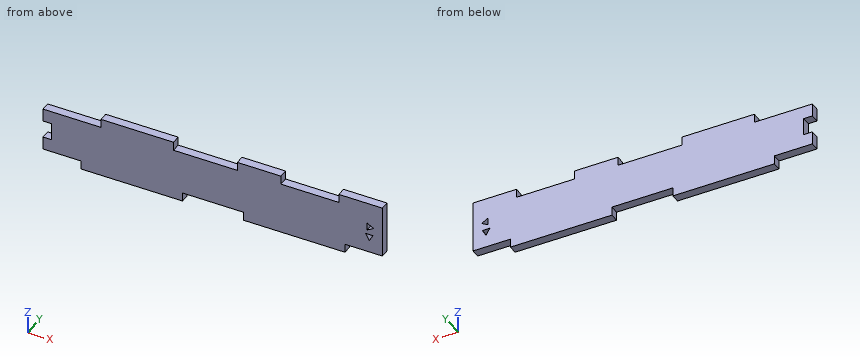
from build123d import *

# Parameters (mm, degrees)
SKETCH1_W                = 117
SKETCH1_H                = 15
BOSS_EXTRUDE1_DEPTH      = 1.5
SKETCH2_W                = 15
SKETCH2_H                = 3
BOSS_EXTRUDE2_DEPTH      = 1.5
SKETCH12_W               = 25
SKETCH12_H               = 3
BOSS_EXTRUDE3_DEPTH      = 1.5
SKETCH13_W               = 35
SKETCH13_H               = 3
BOSS_EXTRUDE4_DEPTH      = 1.5
CUT_EXTRUDE10_DEPTH      = 2.5
CUT_EXTRUDE10_DEPTH_BACK = 2.5
SKETCH16_W               = 3
SKETCH16_H               = 6
CUT_EXTRUDE11_DEPTH      = 2.5
CUT_EXTRUDE11_DEPTH_BACK = 2.5


with BuildPart() as part:
    # Sketch1 → Boss-Extrude1 (new body, symmetric)
    with BuildSketch(Plane(origin=(0, 0, 0), x_dir=(1, 0, 0), z_dir=(0, 1, 0))):
        Rectangle(SKETCH1_W, SKETCH1_H)
    extrude(amount=BOSS_EXTRUDE1_DEPTH, both=True)

    # Sketch2 → Boss-Extrude2 (add, symmetric)
    with BuildSketch(Plane(origin=(0, 0, 0), x_dir=(1, 0, 0), z_dir=(0, 1, 0))):
        with Locations((16, -9)):
            Rectangle(SKETCH2_W, SKETCH2_H)
        with Locations((51, -9)):
            Rectangle(SKETCH2_W, SKETCH2_H)
    extrude(amount=BOSS_EXTRUDE2_DEPTH, both=True)

    # Sketch12 → Boss-Extrude3 (add, symmetric)
    with BuildSketch(Plane(origin=(0, 0, 0), x_dir=(1, 0, 0), z_dir=(0, 1, 0))):
        with Locations((-26, -9)):
            Rectangle(SKETCH12_W, SKETCH12_H)
    extrude(amount=BOSS_EXTRUDE3_DEPTH, both=True)

    # Sketch13 → Boss-Extrude4 (add, symmetric)
    with BuildSketch(Plane(origin=(0, 0, 0), x_dir=(1, 0, 0), z_dir=(0, 1, 0))):
        with Locations((-27.89, 9)):
            Rectangle(SKETCH13_W, SKETCH13_H)
        with Locations((28.11, 9)):
            Rectangle(SKETCH13_W, SKETCH13_H)
    extrude(amount=BOSS_EXTRUDE4_DEPTH, both=True)

    # Sketch15 → Cut-Extrude10 (cut, two sides)
    with BuildSketch(Plane(origin=(0, 0, 0), x_dir=(1, 0, 0), z_dir=(0, 1, 0))) as cut_extrude10_sk:
        Polygon((55.5, -1.799038106), (53.25, -0.5), (53.25, -3.098076211), align=None)
        Polygon((54, 3.202955396), (52.700961894, 0.952955396), (55.299038106, 0.952955396), align=None)
    extrude(amount=CUT_EXTRUDE10_DEPTH, mode=Mode.SUBTRACT)
    extrude(cut_extrude10_sk.sketch, amount=-CUT_EXTRUDE10_DEPTH_BACK, mode=Mode.SUBTRACT)

    # Sketch16 → Cut-Extrude11 (cut, two sides)
    with BuildSketch(Plane(origin=(0, 0, 0), x_dir=(1, 0, 0), z_dir=(0, 1, 0))) as cut_extrude11_sk:
        with Locations((-57, 0)):
            Rectangle(SKETCH16_W, SKETCH16_H)
    extrude(amount=CUT_EXTRUDE11_DEPTH, mode=Mode.SUBTRACT)
    extrude(cut_extrude11_sk.sketch, amount=-CUT_EXTRUDE11_DEPTH_BACK, mode=Mode.SUBTRACT)


solid = part.part
The model under review builds one solid part; all positions refer to its coordinate system, in mm. Coordinates: 2 decimals unless noted, no trailing zeros. Write each loop counter-clockwise with the first axis right and the second up, starting at its lowest first coordinate (ties: lowest second). Pieces come first, ordered by that corner, then holes. Notation, with made-up numbers: (-30.75, 65.25) -> (2.25, 65.25) arc R27 ccw to (2.25, 93.25) -> close; hole circle Ø4 at (66.25, 10.5). An arc over 180 degrees is marked (long way). Answer in a Markdown table with one row per item.
1. We need section B-B, the plane x = 6. State the section outline as (y, z) points, and give its area (3 significant figures).
Answers below:
| item | result |
|---|---|
| outline | (-1.5, -7.5) -> (1.5, -7.5) -> (1.5, 7.5) -> (-1.5, 7.5) -> close |
| area | 45.0 mm^2 |
2. We need section C-C, the plane x = 29.5. State the section outline as (y, z) points, and give its area (3 significant figures).
Answers below:
| item | result |
|---|---|
| outline | (-1.5, -10.5) -> (1.5, -10.5) -> (1.5, 7.5) -> (-1.5, 7.5) -> close |
| area | 54.0 mm^2 |
3. Wall thickness on probe 1 along X at (y, z) = (-0.5, 8.25); probe 2 along Z at (x, y) = (5, 0.6); probe 3 along Z at (x, y) = (47, 0.85): over which ranges is each line inside the solid? List them lowest first. Write a range as [from, to].
Answers below:
| item | result |
|---|---|
| probe 1 | x = [-38.5, -13.5], [8.5, 23.5], [43.5, 58.5] |
| probe 2 | z = [-7.5, 7.5] |
| probe 3 | z = [-7.5, 10.5] |
4. We need section A-A, the plane y = -1. Give the number of separate pieces and of enclosed holes in the cut face, and give its area (3 significant figures).
Answers below:
| item | result |
|---|---|
| separate pieces | 1 |
| enclosed holes | 2 |
| area | 2,110 mm^2 |
5. Clearance check with flat-ended pins moving along their axes: pin 1 Ø1.5 at (y, z) = (-0.5, -9.5) entering from +X; pin 2 Ø0.9 at (x, y) = (54.5, -0.5) entering from -Z; pin 3 Ø0.9 at (y, z) = (-0.5, 9.5) entering from -X. State where each tip first meets the part, or that it passes through.
Answers below:
| item | result |
|---|---|
| pin 1 | stops at x = 45.61 |
| pin 2 | stops at z = -7.5 |
| pin 3 | stops at x = -38.5 |
